CAD build for the part. Positions are in the model's coordinates, mm. Face numbers are marked on the shaded views. Coordinates: 2 decimals unless noted, no trailing zeros. Loops run counter-clockwise (first coordinate to the right, second up) from the corner with the lowest first, then second, coordinate; pieces in that order, holes last. Notation, with made-up numbers: (79.5, -7) -> (90.5, -7) arc R25 ccw to (90.5, 25) -> close; hole circle Ø1 at (-34.5, 9). An arc over 180 degrees is marked (long way). Write each question's results on one line, items separated by ' | '.
```python
from build123d import *

# Parameters (mm, degrees)
SKETCH1_R               = 11
SKETCH1_R_2             = 9
BOSS_EXTRUDE1_DEPTH     = 32
CUT_EXTRUDE1_DEPTH      = 15
CUT_EXTRUDE1_DEPTH_BACK = 9
SKETCH3_R               = 41
BOSS_EXTRUDE2_DEPTH     = 2
FILLET1_R               = 2
SKETCH4_R               = 2.5
CUT_EXTRUDE2_DEPTH      = 2


with BuildPart() as part:
    # Sketch1 → Boss-Extrude1 (new body)
    with BuildSketch(Plane.XY):
        with Locations((0, 3)):
            Circle(SKETCH1_R)
        with Locations((0, 3)):
            Circle(SKETCH1_R_2, mode=Mode.SUBTRACT)
    extrude(amount=-BOSS_EXTRUDE1_DEPTH)

    # Sketch2 → Cut-Extrude1 (cut, two sides)
    with BuildSketch(Plane(origin=(0, 0, 0), x_dir=(1, 0, 0), z_dir=(0, 1, 0))) as cut_extrude1_sk:
        with BuildLine():
            Line((3, 21), (3, 6))
            ThreePointArc((3, 6), (0, 3), (-3, 6))
            Line((-3, 6), (-3, 21))
            ThreePointArc((-3, 21), (0, 24), (3, 21))
        make_face()
    extrude(amount=CUT_EXTRUDE1_DEPTH, mode=Mode.SUBTRACT)
    extrude(cut_extrude1_sk.sketch, amount=-CUT_EXTRUDE1_DEPTH_BACK, mode=Mode.SUBTRACT)

    # Sketch3 → Boss-Extrude2 (add)
    with BuildSketch(Plane.XY):
        Circle(SKETCH3_R)
    extrude(amount=BOSS_EXTRUDE2_DEPTH)

    # Fillet1
    fillet1_edges = [part.edges().sort_by_distance(p)[0] for p in [
        (-11, 3, 0),
    ]]
    fillet(fillet1_edges, radius=FILLET1_R)

    # Sketch4 → Cut-Extrude2 (cut)
    with BuildSketch(Plane.XY.offset(2)):
        with Locations((35.5, 0)):
            Circle(SKETCH4_R)
        with Locations((17.75, -30.743901834)):
            Circle(SKETCH4_R)
        with Locations((-17.75, -30.743901834)):
            Circle(SKETCH4_R)
        with Locations((-35.5, 0)):
            Circle(SKETCH4_R)
        with Locations((-17.75, 30.743901834)):
            Circle(SKETCH4_R)
        with Locations((17.75, 30.743901834)):
            Circle(SKETCH4_R)
    extrude(amount=-CUT_EXTRUDE2_DEPTH, mode=Mode.SUBTRACT)


solid = part.part
```
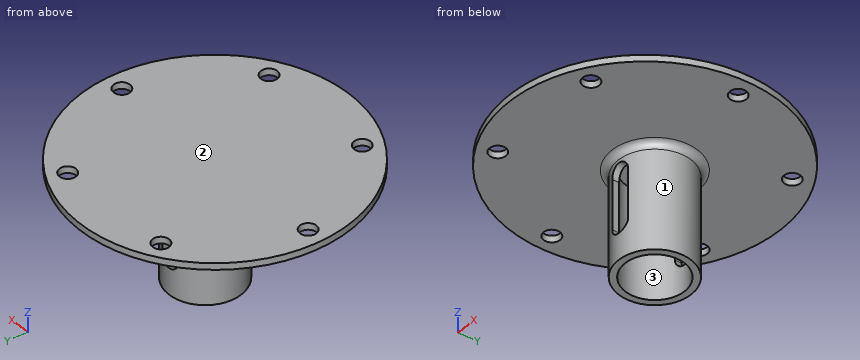
Q1. Cut at C-C on x = 35.5. Write the cut outline in (y, z).
Results are:
outline: (-20.51, 0) -> (-2.5, 0) -> (-2.5, 2) -> (-20.51, 2) -> close; (2.5, 0) -> (20.51, 0) -> (20.51, 2) -> (2.5, 2) -> close
Q2. Drop flat-ended pins along their axis: pin 1 (3 mm diameter, centred on x = 1, y = 1, fed in from -Z); pin 2 (2 mm diameter, centred on x = 8.5, z = -12.5, fed in from +Y); pin 3 (1 mm diameter, centred on y = 12, z = -12, fed in from -X). Give the stop position or say it passes through.
Results are:
pin 1: z = 0 | pin 2: y = 11.05 | pin 3: x = -6.98
Q3. Cut at A-A on z = -11. Write the cut outline in (x, y), and give its area (3 significant figures).
Results are:
outline: (-3, -7.58) -> (-3, -5.49) arc R9 cw to (-3, 11.49) -> (-3, 13.58) arc R11 ccw to start; (3, -7.58) arc R11 ccw to (3, 13.58) -> (3, 11.49) arc R9 cw to (3, -5.49) -> close | area: 101 mm^2
Q4. Wall check: L1, parallel to Y at x = 17, z = 1; L2, parallel to Z at x = 37.5, y = -8; L3, parallel to Y at x = 17.75, z = 0.7. Give the ranges that are in metal, low to high. Write a range as from..to.
Results are:
L1: -37.31..-33.13, -28.36..28.36, 33.13..37.31 | L2: 0..2 | L3: -36.96..-33.24, -28.24..28.24, 33.24..36.96
Q5. Pull direction Y, two halves, no side cores. Call the marked faces 1, 2 and 3: +Y half, -Y half, draft (parallel to the pull), parting line (faces both ways), or undercut.
Results are:
face 1: parting line | face 2: draft | face 3: undercut
Q6. Cut at B-B on x = 0. Write the cut outline in (y, z), and give its area (3 significant figures).
Results are:
outline: (-41, 0) -> (-10, 0) arc R2 cw to (-8, -2) -> (-8, -3) -> (-6, -3) -> (-6, 0) -> (12, 0) -> (12, -3) -> (14, -3) -> (14, -2) arc R2 cw to (16, 0) -> (41, 0) -> (41, 2) -> (-41, 2) -> close; (-8, -32) -> (-6, -32) -> (-6, -24) -> (-8, -24) -> close; (12, -32) -> (14, -32) -> (14, -24) -> (12, -24) -> close | area: 210 mm^2
Q7. Cut at D-D on z = -26. Write the cut outline in (x, y).
Results are:
outline: circle Ø22 at (0, 3); hole circle Ø18 at (0, 3)
